Input: part model. Units: mm. Frame: model coordinates. Face numbers are marked on the shaded views. A direction names the side the tool comes from. Round coordinates to 2 decimals unless told otherwise and drop trailing zeros. Loops run counter-clockwise (first coordinate to the right, second up) from the corner with the lowest first, then second, coordinate; pieces in that order, holes last.
1) Section C-C, the plane y = 0. Return loops of the section in (x, z).
2) Draft query along X for the marked faces 4, 5 and 6. Return one class per face: pulls with the +X half, pulls with the -X half, needs draft (parallel to the pull), parting line crosses it, or undercut.
3) Access query for the marked faces 1, 2 and 3. Directions: +Z, -Z, +X, -X, +Y, -Y. A direction counts if a zero-diameter tool reaches every point of the face in a straight line with its end or side. Return the directions, or none.
4) Section B-B, the plane z = -1.25. Return loops of the section in (x, y).
5) Ray query, line 1 along Y through (x, z) = (4, 1.85); line 2 along Z through (x, y) = (4, 1); line 3 along Z through (x, y) = (6, 3.75). Return the intervals inside material, ascending.
6) Section D-D, the plane x = -4. Return loops of the section in (y, z), and give its area (3 significant figures).
7) First-contact query: pin 1 (2.5 mm diameter, centred on x = -3.5, y = 0.5, fed in from +Z). Flat tip, straight axial feed; report the tip coordinate or a pass-through.
8) Section A-A, the plane z = 2.2. Return loops of the section in (x, y), and give its area (3 significant figures).
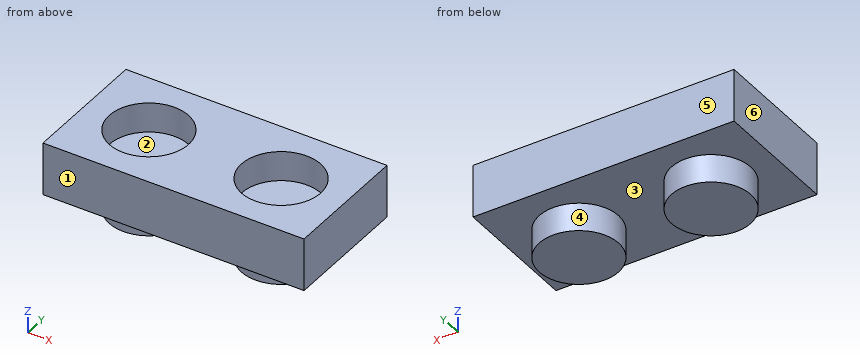
from build123d import *

# Parameters (mm, degrees)
SKETCH_3_W          = 15.8
SKETCH_3_H          = 7.8
EXTRUDE_2_DEPTH     = 3.2
SKETCH_4_R          = 2.4
EXTRUDE_3_DEPTH     = 1.7
SKETCH_5_R          = 2.4
CUT_EXTRUDE_1_DEPTH = 1.8


with BuildPart() as part:
    # Эскиз3 → Бобышка-Вытянуть2 (new body)
    with BuildSketch(Plane.XY):
        Rectangle(SKETCH_3_W, SKETCH_3_H)
    extrude(amount=EXTRUDE_2_DEPTH)

    # Эскиз4 → Бобышка-Вытянуть3 (add)
    with BuildSketch(Plane(origin=(0, 0, 0), x_dir=(-1, 0, 0), z_dir=(0, 0, -1))):
        with Locations((-4, 0)):
            Circle(SKETCH_4_R)
        with Locations((4, 0)):
            Circle(SKETCH_4_R)
    extrude(amount=EXTRUDE_3_DEPTH)

    # Эскиз5 → Вырез-Вытянуть1 (cut)
    with BuildSketch(Plane.XY.offset(3.2)):
        with Locations(Location((-4, 0, 0), (0, 0, 180))):
            Circle(SKETCH_5_R)
        with Locations(Location((4, 0, 0), (0, 0, 180))):
            Circle(SKETCH_5_R)
    extrude(amount=-CUT_EXTRUDE_1_DEPTH, mode=Mode.SUBTRACT)


solid = part.part
Final values:
1. outline: (-7.9, 0) - (-6.4, 0) - (-6.4, -1.7) - (-1.6, -1.7) - (-1.6, 0) - (1.6, 0) - (1.6, -1.7) - (6.4, -1.7) - (6.4, 0) - (7.9, 0) - (7.9, 3.2) - (6.4, 3.2) - (6.4, 1.4) - (1.6, 1.4) - (1.6, 3.2) - (-1.6, 3.2) - (-1.6, 1.4) - (-6.4, 1.4) - (-6.4, 3.2) - (-7.9, 3.2) - close
2. face 4: undercut
2. face 5: needs draft
2. face 6: pulls with the -X half
3. face 1: +Z, -Z, +X, -X, -Y
3. face 2: +Z
3. face 3: -Z
4. outline: circle Ø4.8 at (-4, 0); circle Ø4.8 at (4, 0)
5. line 1: y = -3.9 to -2.4, 2.4 to 3.9
5. line 2: z = -1.7 to 1.4
5. line 3: z = 0 to 3.2
6. outline: (-3.9, 0) - (-2.4, 0) - (-2.4, -1.7) - (2.4, -1.7) - (2.4, 0) - (3.9, 0) - (3.9, 3.2) - (2.4, 3.2) - (2.4, 1.4) - (-2.4, 1.4) - (-2.4, 3.2) - (-3.9, 3.2) - close
6. area: 24.5 mm2
7. pin 1: stops at z = 1.4
8. outline: (-7.9, -3.9) - (7.9, -3.9) - (7.9, 3.9) - (-7.9, 3.9) - close; hole circle Ø4.8 at (-4, 0); hole circle Ø4.8 at (4, 0)
8. area: 87.0 mm2
